Here's how the part is built. I have some questions about the finished solid (model axes, mm). A direction names the side the tool comes from. Round coordinates to 2 decimals unless told otherwise and drop trailing zeros. Order: outer loops, then holes, each group sorted by start corner. A loop starts at its lowest first (then second) coordinate and runs counter-clockwise, first axis right, second up.
```python
from build123d import *

# Parameters (mm, degrees)
SKETCH_1_W           = 32.4
SKETCH_1_H           = 12
SKETCH_1_R           = 1.2
EXTRUDE_1_DEPTH      = 1.5
EXTRUDE_2_DEPTH      = 6.4
EXTRUDE_2_DEPTH_BACK = 19.9
SKETCH_2_W           = 23
SKETCH_2_H           = 12
SKETCH_3_R           = 2.5
EXTRUDE_3_DEPTH      = 5.04


with BuildPart() as part:
    # 草图1 → 凸台-拉伸1 (new body)
    with BuildSketch(Plane.XY):
        Rectangle(SKETCH_1_W, SKETCH_1_H)
        with Locations((-14, 0)):
            Circle(SKETCH_1_R, mode=Mode.SUBTRACT)
        with Locations(Location((14, 0, 0), (0, 0, 180))):
            Circle(SKETCH_1_R, mode=Mode.SUBTRACT)
    extrude(amount=EXTRUDE_1_DEPTH)

    # 草图2 → 凸台-拉伸2 (add, two sides: drawn at the far end of the back side and taken through both)
    with BuildSketch(Plane.XY.offset(1.5).offset(-EXTRUDE_2_DEPTH_BACK)):
        Rectangle(SKETCH_2_W, SKETCH_2_H)
    extrude(amount=EXTRUDE_2_DEPTH + EXTRUDE_2_DEPTH_BACK)

    # 草图3 → 凸台-拉伸3 (add)
    with BuildSketch(Plane.XY.offset(7.9)):
        with Locations((6, 0)):
            Circle(SKETCH_3_R)
    extrude(amount=EXTRUDE_3_DEPTH)


solid = part.part
```
1. I'm going to push flat-ended pins straight in: P1, Ø6, axis at y = 2, z = -12, coming from the +X side; P2, Ø5, axis at x = 14.5, y = -0.5, coming from the +Z side; P3, Ø2, axis at y = 4, z = -8, coming from the -X side; P4, Ø2, axis at x = -4.5, z = 9.5, coming from the +Y side. Where does each tip first touch, or does it pass through?
Evaluation:
P1: stops at x = 11.5
P2: stops at z = 1.5
P3: stops at x = -11.5
P4: passes through
2. If we section it at D-D, the plane y = -4: Write out the boundary of the cut face in (x, z).
Evaluation:
outline: (-16.2, 0) - (-11.5, 0) - (-11.5, -18.4) - (11.5, -18.4) - (11.5, 0) - (16.2, 0) - (16.2, 1.5) - (11.5, 1.5) - (11.5, 7.9) - (-11.5, 7.9) - (-11.5, 1.5) - (-16.2, 1.5) - close
3. If we section it at A-A, the plane x = 14: Write out the boundary of the cut face in (y, z).
Evaluation:
outline: (-6, 0) - (-1.2, 0) - (-1.2, 1.5) - (-6, 1.5) - close; (1.2, 0) - (6, 0) - (6, 1.5) - (1.2, 1.5) - close
4. If we section it at C-C, the plane x = 4: Write out the boundary of the cut face in (y, z), and give its area (3 significant figures).
Evaluation:
outline: (-6, -18.4) - (6, -18.4) - (6, 7.9) - (1.5, 7.9) - (1.5, 12.94) - (-1.5, 12.94) - (-1.5, 7.9) - (-6, 7.9) - close
area: 331 mm2
5. On a 3-axis mill with a long thin cutter (end or side, diameter ignored), from which of +Z, -Z, +X, -X, +Y, -Y can I reach the whole of each face in a straight line? I mean faces 4 (the flat face through (-13.9, 1.4, 0)), 5 (the flat face through (13.8, 1.4, 0)), 6 (the flat face through (11.5, 0, 5)). Say none if no direction works.
Evaluation:
face 4: -Z, -X, +Y, -Y
face 5: -Z, +X, +Y, -Y
face 6: +Z, +X, +Y, -Y
6. I need wall thicknesses on probe 1 along Y at (x, z) = (-14, 1.05); probe 2 along Z at (x, y) = (13, 2.75); probe 3 along X at (y, z) = (-2.75, 2.5). Which ranges of each line are inside material? Lowest first, please.
Evaluation:
probe 1: y = -6 to -1.2, 1.2 to 6
probe 2: z = 0 to 1.5
probe 3: x = -11.5 to 11.5
7. If we mould it in two halves opening along Y, with no side actions, what happens to faces 1 (the cylindrical face through (8.385, 0.751, 10.385)), 2 (the flat face through (0, 0, 7.9)), 3 (the cylindrical face through (-12.855, 0.36, 0.74))? For each: released by +Y, released by -Y, zero draft, split by the parting line, or undercut.
Evaluation:
face 1: split by the parting line
face 2: zero draft
face 3: undercut
8. If we section it at B-B, the plane y = 0: Write out the boundary of the cut face in (x, z).
Evaluation:
outline: (-16.2, 0) - (-15.2, 0) - (-15.2, 1.5) - (-16.2, 1.5) - close; (-12.8, 0) - (-11.5, 0) - (-11.5, -18.4) - (11.5, -18.4) - (11.5, 0) - (12.8, 0) - (12.8, 1.5) - (11.5, 1.5) - (11.5, 7.9) - (8.5, 7.9) - (8.5, 12.94) - (3.5, 12.94) - (3.5, 7.9) - (-11.5, 7.9) - (-11.5, 1.5) - (-12.8, 1.5) - close; (15.2, 0) - (16.2, 0) - (16.2, 1.5) - (15.2, 1.5) - close
